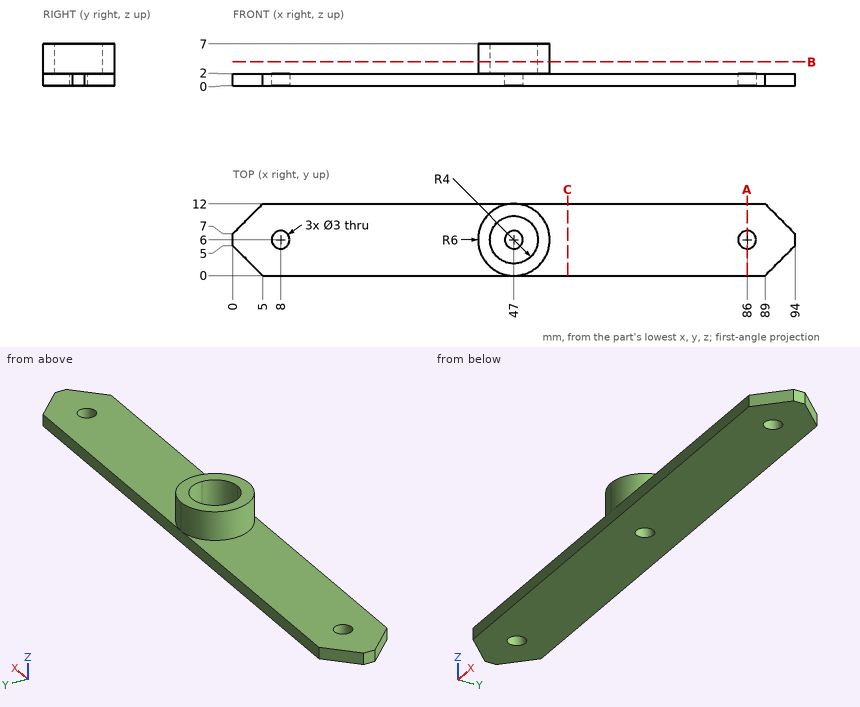
Print and shaded views of the part. All mm, measured from the part's lowest x, y and z. Give positions to 0.01 mm unless a question says otherwise; leave off trailing zeros. Write each loop counter-clockwise with the first axis right and the second up, starting at its lowest first coordinate (ties: lowest second). Pieces come first, ordered by that corner, then holes. Notation, with made-up numbers: (32.25, -35.5) -> (91.25, -35.5) arc R21 ccw to (91.25, -21.5) -> close; hole circle Ø10 at (-32.75, 18). An arc over 180 degrees is marked (long way). Write each question's results on one line, items separated by ' | '.
1. Cut at B-B, the plane z = 4. Write the cut outline in (x, y).
Geometry check:
outline: circle Ø12 at (47, 6); hole circle Ø8 at (47, 6)
2. Drop flat-ended pins along their axis: P1, Ø5, axis at x = 80.5, y = 10.5, coming from the +Z side; P2, Ø1.5, axis at y = 1.5, z = 2.5, coming from the +X side. Give the stop position or say it passes through.
Geometry check:
P1: z = 2 | P2: x = 91.06
3. Cut at A-A, the plane x = 86. Write the cut outline in (y, z).
Geometry check:
outline: (0, 0) -> (4.5, 0) -> (4.5, 2) -> (0, 2) -> close; (7.5, 0) -> (12, 0) -> (12, 2) -> (7.5, 2) -> close
4. Wall check: probe 1 along Y at (x, z) = (8, 1.25); probe 2 along Z at (x, y) = (37.5, 2.75); probe 3 along X at (y, z) = (7, 5.5). Give the ranges that are in metal, low to high. Write a range as [from, to].
Geometry check:
probe 1: [0, 4.5], [7.5, 12] | probe 2: [0, 2] | probe 3: [41.08, 43.13], [50.87, 52.92]
5. Cut at C-C, the plane x = 56. Write the cut outline in (y, z), then the cut area to 3 significant figures.
Geometry check:
outline: (0, 0) -> (12, 0) -> (12, 2) -> (0, 2) -> close | area: 24.0 mm²
